Build history of the part. All positions in model axes, mm. Face numbers are marked on the shaded views. Coordinates: 2 decimals unless noted, no trailing zeros. Write each question's results on one line, items separated by ' | '. Start each with the question number.
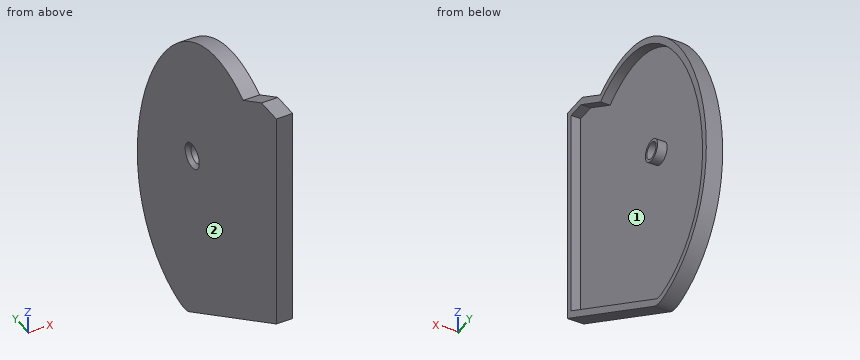
from build123d import *

# Parameters (mm, degrees)
SKETCH1_R                                         = 1.27
BOSS_EXTRUDE1_DEPTH                               = 4.9276
SHELL1_T                                          = -2.032
CSK_FOR_0_FLAT_HEAD_MACHINE_SCREW_100_D           = 5.08
CSK_FOR_0_FLAT_HEAD_MACHINE_SCREW_100_CSINK_D     = 7.62
CSK_FOR_0_FLAT_HEAD_MACHINE_SCREW_100_CSINK_ANGLE = 100


with BuildPart() as part:
    # Sketch1 → Boss-Extrude1 (new body)
    with BuildSketch(Plane(origin=(0, 0, 0), x_dir=(0, 0, -1), z_dir=(1, 0, 0))):
        with BuildLine():
            Line((0, 0), (-67.7418, 0))
            Line((-67.7418, 0), (-67.7418, 7.990379))
            Line((-67.7418, 7.990379), (-62.052733, 17.844133))
            add(Edge.make_bspline(
                [(-62.052733, 17.844133), (-83.520452, 52.181699), (-7.196896, 94.452135), (26.093729, 59.797721), (28.153169, 48.762718), (27.0383, 46.831709)],
                knots=[0, 0, 0, 0, 0.772335, 0.951961, 1, 1, 1, 1], degree=3))
            Line((27.0383, 46.831709), (0, 0))
        make_face()
        with Locations((-25.4, 45.3644)):
            Circle(SKETCH1_R, mode=Mode.SUBTRACT)
    extrude(amount=BOSS_EXTRUDE1_DEPTH)

    # Shell1
    shell1_openings = [part.faces().sort_by_distance(p)[0] for p in [
        (4.9276, 17.432002, 25.190503),
    ]]
    offset(amount=SHELL1_T, openings=shell1_openings, kind=Kind.INTERSECTION)

    # CSK for #0 Flat Head Machine Screw (100)2 (through all)
    with Locations(Plane.ZY):
        with Locations((25.4, 45.3644)):
            CounterSinkHole(CSK_FOR_0_FLAT_HEAD_MACHINE_SCREW_100_D / 2, CSK_FOR_0_FLAT_HEAD_MACHINE_SCREW_100_CSINK_D / 2, counter_sink_angle=CSK_FOR_0_FLAT_HEAD_MACHINE_SCREW_100_CSINK_ANGLE)


solid = part.part
Item 1: Pull direction Z, two halves, no side cores. Call the marked faces 1 and 2: released by +Z, released by -Z, zero draft, split by the parting line, or undercut.
Item 2: Flat gauge pins, fed straight in: P1, Ø1.4, axis at x = 4, y = 5.5, coming from the -Z side; P2, Ø5, axis at y = 42, z = -13.5, coming from the -X side; P3, Ø3, axis at y = 22, z = 21.5, coming from the +X side. Where does each tip first touch, or does it go through?
Item 3: Probe probe 1 along Y at (x, z) = (3.4, 28); probe 2 along Y at (x, z) = (3.35, 25.4); probe 3 along X at (y, z) = (32, 16). List the from-to ranges inside material, lowest first.
Resolved:
1) face 1: undercut | face 2: zero draft
2) P1: z = -3.58 | P2: x = 0 | P3: x = 2.03
3) probe 1: 0 to 2.03, 43.33 to 47.4, 69.41 to 71.55 | probe 2: 0 to 2.03, 42.06 to 42.82, 47.9 to 48.67, 70.22 to 72.33 | probe 3: 0 to 2.03
